from build123d import *
from build123d.topology import SkipClean

# Parameters (mm, degrees)
SKETCH1_W           = 46
SKETCH1_H           = 2
BOSS_EXTRUDE1_DEPTH = 22
SKETCH2_W           = 29.75
SKETCH2_H           = 22
BOSS_EXTRUDE2_DEPTH = 13
SKETCH3_W           = 27.75
SKETCH3_H           = 11
CUT_EXTRUDE1_DEPTH  = 22
SKETCH4_R           = 4.25
CUT_EXTRUDE2_DEPTH  = 1
SKETCH5_R           = 3.5
CUT_EXTRUDE3_DEPTH  = 1
BOSS_EXTRUDE4_START = 6
BOSS_EXTRUDE4_DEPTH = 6
SKETCH20_W          = 11
SKETCH20_H          = 2
BOSS_EXTRUDE8_DEPTH = 3
SKETCH6_W           = 4
SKETCH6_H           = 20
CUT_EXTRUDE4_DEPTH  = 35.380226875
SKETCH25_W          = 2
SKETCH25_H          = 1.75
CUT_EXTRUDE7_DEPTH  = 47.707199659
SKETCH26_R          = 0.75
CUT_EXTRUDE8_DEPTH  = 13
BOSS_EXTRUDE3_DEPTH = 2
SKETCH13_R          = 3.25
CUT_EXTRUDE5_DEPTH  = 1
SKETCH14_R          = 2.5
CUT_EXTRUDE6_DEPTH  = 1
BOSS_EXTRUDE6_START = 5
BOSS_EXTRUDE6_DEPTH = 5


with BuildPart() as part:
    # Sketch1 → Boss-Extrude1 (new body)
    with BuildSketch(Plane.XY):
        Rectangle(SKETCH1_W, SKETCH1_H)
    extrude(amount=-BOSS_EXTRUDE1_DEPTH)

    # Sketch2 → Boss-Extrude2 (add)
    with BuildSketch(Plane(origin=(0, 1, 0), x_dir=(1, 0, 0), z_dir=(0, 1, 0))):
        with Locations((8.125, 11)):
            Rectangle(SKETCH2_W, SKETCH2_H)
    extrude(amount=BOSS_EXTRUDE2_DEPTH)

    # Sketch3 → Cut-Extrude1 (cut)
    with BuildSketch(Plane.XY):
        with Locations((9.125, 6.5)):
            Rectangle(SKETCH3_W, SKETCH3_H)
    extrude(amount=-CUT_EXTRUDE1_DEPTH, mode=Mode.SUBTRACT)

    # Sketch4 → Cut-Extrude2 (cut)
    with BuildSketch(Plane(origin=(0, 1, 0), x_dir=(1, 0, 0), z_dir=(0, 1, 0))):
        with Locations(Location((-17.75, 11, 0), (0, 0, 180))):
            Circle(SKETCH4_R)
    extrude(amount=-CUT_EXTRUDE2_DEPTH, mode=Mode.SUBTRACT)

    # Sketch5 → Cut-Extrude3 (cut)
    with BuildSketch(Plane(origin=(0, 0, 0), x_dir=(1, 0, 0), z_dir=(0, 1, 0))):
        with Locations(Location((-17.75, 11, 0), (0, 0, 180))):
            Circle(SKETCH5_R)
    extrude(amount=-CUT_EXTRUDE3_DEPTH, mode=Mode.SUBTRACT)

    # Sketch16 → Boss-Extrude4 (add)
    with SkipClean():  # the faces are left unmerged after this step: merging them gives an invalid solid
        with BuildSketch(Plane(origin=(0, 1, 0), x_dir=(1, 0, 0), z_dir=(0, 1, 0)).offset(BOSS_EXTRUDE4_START)):
            with BuildLine():
                Line((-18.75, 6.86932209), (-18.75, 5.86932209))
                Line((-18.75, 5.86932209), (-16.75, 5.86932209))
                Line((-16.75, 5.86932209), (-16.75, 6.86932209))
                ThreePointArc((-16.75, 6.86932209), (-17.75, 6.75), (-18.75, 6.86932209))
            make_face()
        boss_extrude4 = extrude(amount=-BOSS_EXTRUDE4_DEPTH)

    # Sketch20 → Boss-Extrude8 (add)
    with SkipClean():  # the faces are left unmerged after this step: merging them gives an invalid solid
        with BuildSketch(Plane(origin=(0, 1, 0), x_dir=(1, 0, 0), z_dir=(0, 1, 0))):
            with Locations((-10.25, 15.84)):
                Rectangle(SKETCH20_W, SKETCH20_H)
        boss_extrude8 = extrude(amount=-BOSS_EXTRUDE8_DEPTH)

    # Sketch6 → Cut-Extrude4 (cut, through all)
    with SkipClean():  # the faces are left unmerged after this step: merging them gives an invalid solid
        with BuildSketch(Plane(origin=(0, 1, 0), x_dir=(1, 0, 0), z_dir=(0, 1, 0))):
            with Locations((-10.75, 11)):
                Rectangle(SKETCH6_W, SKETCH6_H)
        cut_extrude4 = extrude(amount=-CUT_EXTRUDE4_DEPTH, mode=Mode.SUBTRACT)

    # Sketch25 → Cut-Extrude7 (cut, through all)
    with SkipClean():  # the faces are left unmerged after this step: merging them gives an invalid solid
        with BuildSketch(Plane.ZY.offset(15.75)):
            with Locations((-15.84, -1.125)):
                Rectangle(SKETCH25_W, SKETCH25_H)
        cut_extrude7 = extrude(amount=CUT_EXTRUDE7_DEPTH, mode=Mode.SUBTRACT)

    # Sketch26 → Cut-Extrude8 (cut)
    with SkipClean():  # the faces are left unmerged after this step: merging them gives an invalid solid
        with BuildSketch(Plane.ZY.offset(15.75)):
            with Locations(Location((-15.84, -1, 0), (0, 0, 270))):
                Circle(SKETCH26_R)
        cut_extrude8 = extrude(amount=-CUT_EXTRUDE8_DEPTH, mode=Mode.SUBTRACT)

    # Mirror8: Boss-Extrude4, Boss-Extrude8, Cut-Extrude4, Cut-Extrude7, Cut-Extrude8 across plane
    with SkipClean():  # the faces are left unmerged after this step: merging them gives an invalid solid
        add(boss_extrude4.mirror(Plane.XY.offset(-11)))
        add(boss_extrude8.mirror(Plane.XY.offset(-11)))
        add(cut_extrude4.mirror(Plane.XY.offset(-11)), mode=Mode.SUBTRACT)
        add(cut_extrude7.mirror(Plane.XY.offset(-11)), mode=Mode.SUBTRACT)
        add(cut_extrude8.mirror(Plane.XY.offset(-11)), mode=Mode.SUBTRACT)

    # Sketch12 → Boss-Extrude3 (add)
    with SkipClean():  # the faces are left unmerged after this step: merging them gives an invalid solid
        with BuildSketch(Plane(origin=(0, 14, 0), x_dir=(1, 0, 0), z_dir=(0, 1, 0))):
            Polygon((23, 22), (18, 22), (18, 26), (32.25, 26), (32.25, 11), (25.5, 11), (25.5, 24), (23, 24), align=None)
        boss_extrude3 = extrude(amount=-BOSS_EXTRUDE3_DEPTH)

    # Sketch13 → Cut-Extrude5 (cut)
    with SkipClean():  # the faces are left unmerged after this step: merging them gives an invalid solid
        with BuildSketch(Plane(origin=(0, 14, 0), x_dir=(1, 0, 0), z_dir=(0, 1, 0))):
            with Locations((28.875, 11)):
                Circle(SKETCH13_R)
        cut_extrude5 = extrude(amount=-CUT_EXTRUDE5_DEPTH, mode=Mode.SUBTRACT)

    # Sketch14 → Cut-Extrude6 (cut)
    with SkipClean():  # the faces are left unmerged after this step: merging them gives an invalid solid
        with BuildSketch(Plane(origin=(0, 13, 0), x_dir=(1, 0, 0), z_dir=(0, 1, 0))):
            with Locations((28.875, 11)):
                Circle(SKETCH14_R)
        cut_extrude6 = extrude(amount=-CUT_EXTRUDE6_DEPTH, mode=Mode.SUBTRACT)

    # Sketch18 → Boss-Extrude6 (add)
    with SkipClean():  # the faces are left unmerged after this step: merging them gives an invalid solid
        with BuildSketch(Plane(origin=(0, 14, 0), x_dir=(1, 0, 0), z_dir=(0, 1, 0)).offset(BOSS_EXTRUDE6_START)):
            with BuildLine():
                Line((29.875, 14.092329219), (29.875, 15.092329219))
                Line((29.875, 15.092329219), (27.875, 15.092329219))
                Line((27.875, 15.092329219), (27.875, 14.092329219))
                ThreePointArc((27.875, 14.092329219), (28.875, 14.25), (29.875, 14.092329219))
            make_face()
        boss_extrude6 = extrude(amount=-BOSS_EXTRUDE6_DEPTH)

    # Mirror3: Boss-Extrude3, Cut-Extrude5, Cut-Extrude6, Boss-Extrude6 across plane
    with SkipClean():  # the faces are left unmerged after this step: merging them gives an invalid solid
        add(boss_extrude3.mirror(Plane.XY.offset(-11)))
        add(cut_extrude5.mirror(Plane.XY.offset(-11)), mode=Mode.SUBTRACT)
        add(cut_extrude6.mirror(Plane.XY.offset(-11)), mode=Mode.SUBTRACT)
        add(boss_extrude6.mirror(Plane.XY.offset(-11)))


solid = part.part
Source: CAD feature listing. Evaluate the final solid. Frame: model axes, mm. A direction names the side the tool comes from. Coordinates: 2 decimals unless noted, no trailing zeros. Loops run counter-clockwise (first coordinate to the right, second up) from the corner with the lowest first, then second, coordinate; pieces in that order, holes last. Notation, with made-up numbers: M 68,48.25 L 99,48.25 A26 cw 99,62.25 Z; hole C -2.5,-12 d3. An arc over 180 degrees is marked long. Answer in a Markdown table with one row per item.
Q1. Ray query, probe 1 along X at (y, z) = (0.4, -11); probe 2 along X at (y, z) = (13.5, -3.5); probe 3 along Y at (x, z) = (-6.8, -15.84). Return the intervals inside material, ascending. Write a range as from..to.
Answers below:
| item | result |
|---|---|
| probe 1 | x = -23..-22, -13.5..-12.75, -8.75..23 |
| probe 2 | x = -6.75..23, 25.5..32.25 |
| probe 3 | y = -2..-1.75, -0.25..1 |
Q2. Section A-A on z = -17.5. Return the cut outline in (x, y).
Answers below:
| item | result |
|---|---|
| outline | M -23,-1 L -12.75,-1 L -12.75,1 L -23,1 Z; M -8.75,-1 L 23,-1 L 23,1 L -4.75,1 L -4.75,12 L 23,12 L 23,14 L -6.75,14 L -6.75,1 L -8.75,1 Z; M 25.5,12 L 32.25,12 L 32.25,14 L 25.5,14 Z |
Q3. Draft query along X for faces 1 (the flat face through (-14.3, -1.5, -5.16)), 2 (the flat face through (-16.75, 4, -6.4)), 3 (the flat face through (23, 0, -11)). Return one class per face: pulls with the +X half, pulls with the -X half, needs draft (parallel to the pull), parting line crosses it, or undercut.
Answers below:
| item | result |
|---|---|
| face 1 | needs draft |
| face 2 | undercut |
| face 3 | pulls with the +X half |
Q4. Section D-D on x = 14.5. Return the cut outline in (y, z).
Answers below:
| item | result |
|---|---|
| outline | M -1,-22 L 1,-22 L 1,0 L -1,0 Z; M 12,-22 L 14,-22 L 14,0 L 12,0 Z |
Q5. First-contact query: pin 1 (1.1 mm diameter, centred on y = 4.5, z = -6.5, fed in from +X); pin 2 (0.8 mm diameter, centred on y = -1.5, z = -6, fed in from -X); pin 3 (0.6 mm diameter, centred on x = -14, z = -6.5, fed in from +Y). Flat tips, straight axial feed; report the tip coordinate or a pass-through.
Answers below:
| item | result |
|---|---|
| pin 1 | stops at x = -4.75 |
| pin 2 | stops at x = -15.75 |
| pin 3 | stops at y = 1 |
Q6. Section B-B on y = 2.75. Return the cut outline in (x, z).
Answers below:
| item | result |
|---|---|
| outline | M -18.75,-16.13 L -16.75,-16.13 L -16.75,-15.13 A4.25 cw -18.75,-15.13 Z; M -18.75,-6.87 A4.25 cw -16.75,-6.87 L -16.75,-5.87 L -18.75,-5.87 Z; M -6.75,-22 L -4.75,-22 L -4.75,0 L -6.75,0 Z |
Q7. Section C-C on x = -17.75. Return the cut outline in (y, z), plus the area to 3 significant figures.
Answers below:
| item | result |
|---|---|
| outline | M -1,-22 L 1,-22 L 1,-16.13 L 7,-16.13 L 7,-15.25 L 0,-15.25 L 0,-14.5 L -1,-14.5 L -1,-14.84 L -0.25,-14.84 L -0.25,-16.84 L -1,-16.84 Z; M -1,-7.5 L 0,-7.5 L 0,-6.75 L 7,-6.75 L 7,-5.87 L 1,-5.87 L 1,0 L -1,0 L -1,-5.16 L -0.25,-5.16 L -0.25,-7.16 L -1,-7.16 Z |
| area | 36.1 mm^2 |
Q8. Set-up query: faces 4 (the flat face through (-18.75, 4, -6.4)), 5 (the flat face through (29.875, 16.5, -14.6)), 6 (the flat face through (-6.8, -1.5, -14.84)). Return all of +Z, -Z, +X, -X, +Y, -Y with unobstructed straight access to the full face (end or side cutting, diameter ignored); none if empty.
Answers below:
| item | result |
|---|---|
| face 4 | +Z, -Z, -X, +Y |
| face 5 | +Z, -Z, +X, +Y |
| face 6 | +X, -X, -Y |
